from build123d import *

# Parameters (mm, degrees)
CYLINDER001_R     = 62
CYLINDER001_DEPTH = 24
PAD004_DEPTH      = 128


with BuildPart() as cylinder001:
    # Cylinder001 → Cylinder001 (new body)
    with BuildSketch(Plane.XZ.offset(-12)):
        Circle(CYLINDER001_R)
    extrude(amount=CYLINDER001_DEPTH)


with BuildPart() as body004:
    # Sketch004 → Pad004 (new body)
    with BuildSketch(Plane.YZ):
        Polygon((0, 0), (12, 0), (5, -294), (0, -294), align=None)
    extrude(amount=PAD004_DEPTH)


with BuildPart() as body004_1:
    # Body004 placement: moved
    add(body004.part.moved(Location((0, 0, 210))))


with BuildPart() as obj1:
    # Part__Mirroring007: instance of Body004
    add(body004_1.part.mirror(Plane(origin=(0, 0, 0), x_dir=(1, 0, 0), z_dir=(0, 1, 0))))

    # Fusion015: union Body004
    add(body004_1.part)


with BuildPart() as obj1_1:
    # Fusion015 placement: moved
    add(obj1.part.moved(Location((-64, 0, 0))))

    # Common001: intersect Cylinder001
    add(cylinder001.part, mode=Mode.INTERSECT)


solid = obj1_1.part
The model under review builds one solid part; all positions refer to its coordinate system, in mm. Give positions to 0.01 mm unless a question says otherwise; leave off trailing zeros. Order: outer loops, then holes, each group sorted by start corner. A loop starts at its lowest first (then second) coordinate and runs counter-clockwise, first axis right, second up. Notation, with made-up numbers: M 32.5,72.25 L 54.5,72.25 A34 ccw 54.5,109.25 Z; hole C 64,33 d3. An arc over 180 degrees is marked long. Answer in a Markdown table with one row per item. Add a question column.
1. Add section B-B on x = 0. State the section outline as (y, z) points.
2. For pin 1 Ø1.5 at (x, y) = (-24, -6.5) entering from +Z; pin 2 Ø5 at (y, z) = (1.5, 41.5) entering from +X; pin 3 Ø8 at (x, z) = (27.5, -42.5) entering from +Y, all flat-tipped, find the tip position at first contact; note any pin that passes through.
3. To check wall thickness, follow line 1 along Z through (x, y) = (-0.5, -0.5); line 2 along X through (y, z) = (3.5, 55.5); line 3 along Y through (x, z) = (-25, -13.5). State the ranges of each line that lie inside material, in increasing order.
4. Add section A-A on z = 0. State the section outline as (x, y) points, plus the area to 3 significant figures.
5. Add section C-C on y = -0.75. State the section outline as (x, z) points.
The answers:
| question | item | result |
|---|---|---|
| 1 | outline | M -8.48,62 L -5.52,-62 L 5.52,-62 L 8.48,62 Z |
| 2 | pin 1 | z = 57.48 |
| 2 | pin 2 | x = 48.2 |
| 2 | pin 3 | y = 6.08 |
| 3 | line 1 | -62 to 62 |
| 3 | line 2 | -27.64 to 27.64 |
| 3 | line 3 | -6.68 to 6.68 |
| 4 | outline | M -62,-7 L 62,-7 L 62,7 L -62,7 Z |
| 4 | area | 1,740 mm2 |
| 5 | outline | C 0,0 d124 |
